For this review, take the finished solid that the model builds, in its own axes (mm). Face numbers are marked on the shaded views. A direction names the side the tool comes from. Coordinates: 2 decimals unless noted, no trailing zeros. Write each loop counter-clockwise with the first axis right and the second up, starting at its lowest first coordinate (ties: lowest second). Pieces come first, ordered by that corner, then holes.
1) Mouldability with a two-part tool opening along Z and no side actions: class the marked faces 1, 2 and 3 as pulls with the +Z half, pulls with the -Z half, needs draft (parallel to the pull), parting line crosses it, or undercut.
2) We need section C-C on x = -17. Write out the cut boundary in (y, z) (3 decimals), then the cut area to 3 significant figures.
3) We need section B-B on y = 33. Write out the cut boundary in (x, z), then the cut area to 3 significant figures.
4) Insertion check: P1, Ø1.5, axis at y = 12, z = 9, coming from the -X side; P2, Ø2, axis at y = 35.55, z = -10.55, coming from the +X side; P3, Ø4, axis at x = -17, z = 17, coming from the -Y side; P4, Ø1, axis at x = -2.5, z = -7.5, coming from the +Y side. Each pin has a flat end and moves straight along its axis. Give the tip position at first contact, or say it passes through.
5) We need section D-D on z = 8. Write out the cut boundary in (x, y).
6) We need section A-A on z = 0. Write out the cut boundary in (x, y), then the cut area to 3 significant figures.
7) For the marked faces 4 and 5, list the 3-axis set-ups (+Z, -Z, +X, -X, +Y, -Y) from which the entire face can be reached by the end or side of a thin tool; tool diameter is ignored.
8) To check wall thickness, follow line 1 along X through (y, z) = (2, 17); line 2 along Y through (x, z) = (10.5, -1); line 3 along X through (y, z) = (21.5, 15.5). State the ranges of each line that lie inside material, in increasing order.
from build123d import *

# Parameters (mm, degrees)
SKETCH1_W                      = 40
SKETCH1_H                      = 40
BOSS_EXTRUDE1_DEPTH            = 5
BOSS_EXTRUDE2_START            = 20
SKETCH2_W                      = 40
SKETCH2_H                      = 45
BOSS_EXTRUDE2_DEPTH            = 5
FILLET1_R                      = 10
FILLET2_R                      = 10
FILLET3_R                      = 5
SKETCH3_R                      = 10
CUT_EXTRUDE1_DEPTH             = 5
M3_CLEARANCE_HOLE1_D           = 3.4
M3_CLEARANCE_HOLE1_CSINK_D     = 3.45
M3_CLEARANCE_HOLE1_CSINK_ANGLE = 90
CIRPATTERN1_COUNT              = 4
M3_CLEARANCE_HOLE2_D           = 3.4
M3_CLEARANCE_HOLE2_CSINK_D     = 3.45
M3_CLEARANCE_HOLE2_CSINK_ANGLE = 90
CIRPATTERN2_COUNT              = 4


with BuildPart() as part:
    # Sketch1 → Boss-Extrude1 (new body)
    with BuildSketch(Plane(origin=(0, 0, 0), x_dir=(1, 0, 0), z_dir=(0, 1, 0))):
        Rectangle(SKETCH1_W, SKETCH1_H)
    extrude(amount=BOSS_EXTRUDE1_DEPTH)

    # Sketch2 → Boss-Extrude2 (add)
    with BuildSketch(Plane(origin=(0, 0, 0), x_dir=(0, 0, -1), z_dir=(1, 0, 0)).offset(BOSS_EXTRUDE2_START)):
        with Locations((0, 22.5)):
            Rectangle(SKETCH2_W, SKETCH2_H)
    extrude(amount=BOSS_EXTRUDE2_DEPTH)

    # Fillet1
    fillet1_edges = [part.edges().sort_by_distance(p)[0] for p in [
        (22.5, 45, 20),
    ]]
    fillet(fillet1_edges, radius=FILLET1_R)

    # Fillet2
    fillet2_edges = [part.edges().sort_by_distance(p)[0] for p in [
        (22.5, 45, -20),
    ]]
    fillet(fillet2_edges, radius=FILLET2_R)

    # Fillet3
    fillet3_edges = [part.edges().sort_by_distance(p)[0] for p in [
        (25, 0, 0),
    ]]
    fillet(fillet3_edges, radius=FILLET3_R)

    # Sketch3 → Cut-Extrude1 (cut)
    with BuildSketch(Plane.ZY.offset(-20)):
        with Locations((0, 25)):
            Circle(SKETCH3_R)
    extrude(amount=-CUT_EXTRUDE1_DEPTH, mode=Mode.SUBTRACT)

    # M3 Clearance Hole1 (through all)
    with Locations(Plane(origin=(25, 0, 0), x_dir=(0, 0, -1), z_dir=(1, 0, 0))):
        with Locations((-10.553493254, 35.553493254)):
            m3_clearance_hole1 = CounterSinkHole(M3_CLEARANCE_HOLE1_D / 2, M3_CLEARANCE_HOLE1_CSINK_D / 2, counter_sink_angle=M3_CLEARANCE_HOLE1_CSINK_ANGLE)

    # CirPattern1: M3 Clearance Hole1 ×4 about axis
    cirpattern1_axis = Axis((0, 25, 0), (1, 0, 0))
    for i in range(1, CIRPATTERN1_COUNT):
        add(m3_clearance_hole1.rotate(cirpattern1_axis, i * 360 / CIRPATTERN1_COUNT), mode=Mode.SUBTRACT)

    # M3 Clearance Hole2 (through all)
    with Locations(Plane(origin=(0, 5, 0), x_dir=(1, 0, 0), z_dir=(0, 1, 0))):
        with Locations((-17, -17)):
            m3_clearance_hole2 = CounterSinkHole(M3_CLEARANCE_HOLE2_D / 2, M3_CLEARANCE_HOLE2_CSINK_D / 2, counter_sink_angle=M3_CLEARANCE_HOLE2_CSINK_ANGLE)

    # CirPattern2: M3 Clearance Hole2 ×4 about axis
    cirpattern2_axis = Axis((0.09990837, 0, -0.09990837), (0, 1, 0))
    for i in range(1, CIRPATTERN2_COUNT):
        add(m3_clearance_hole2.rotate(cirpattern2_axis, i * 360 / CIRPATTERN2_COUNT), mode=Mode.SUBTRACT)


solid = part.part
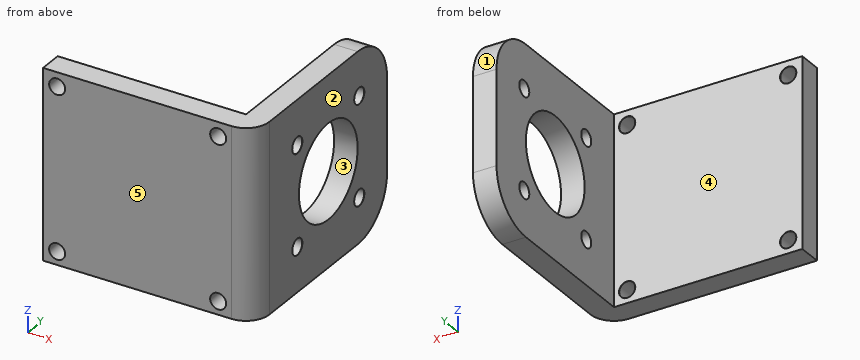
Result:
1. face 1: pulls with the +Z half
1. face 2: needs draft
1. face 3: undercut
2. outline: (0, -20) - (5, -20) - (5, -18.925) - (4.975, -18.9) - (0, -18.9) - close; (0, -15.5) - (4.975, -15.5) - (5, -15.475) - (5, 15.275) - (4.975, 15.3) - (0, 15.3) - close; (0, 18.7) - (4.975, 18.7) - (5, 18.725) - (5, 20) - (0, 20) - close
2. area: 166 mm2
3. outline: (20, -20) - (25, -20) - (25, -6) - (20, -6) - close; (20, 6) - (25, 6) - (25, 20) - (20, 20) - close
3. area: 140 mm2
4. P1: stops at x = 20
4. P2: passes through
4. P3: stops at y = 0
4. P4: stops at y = 5
5. outline: (-20, 0) - (20, 0) arc R5 ccw to (25, 5) - (25, 19) - (20, 19) - (20, 5) - (-20, 5) - close; (20, 31) - (25, 31) - (25, 45) - (20, 45) - close
6. outline: (-20, 0) - (20, 0) arc R5 ccw to (25, 5) - (25, 15) - (20, 15) - (20, 5) - (-20, 5) - close; (20, 35) - (25, 35) - (25, 45) - (20, 45) - close
6. area: 320 mm2
7. face 4: +Z, -Z, -X, +Y
7. face 5: +Z, -Z, +X, -X, -Y
8. line 1: x = -20 to -18.7, -15.3 to 15.5, 18.9 to 24
8. line 2: y = 0 to 5
8. line 3: x = 20 to 25
